from build123d import *

# Parameters (mm, degrees)
BOSS_EXTRUDE1_DEPTH = 4
BOSS_EXTRUDE2_DEPTH = 4
BOSS_EXTRUDE3_DEPTH = 4
SKETCH5_R           = 3
CUT_EXTRUDE2_DEPTH  = 4
SKETCH6_R           = 3
CUT_EXTRUDE3_DEPTH  = 4
SKETCH7_R           = 3
CUT_EXTRUDE4_DEPTH  = 4


with BuildPart() as part:
    # Sketch1 → Boss-Extrude1 (new body)
    with BuildSketch(Plane(origin=(0, 0, 0), x_dir=(1, 0, 0), z_dir=(0, 1, 0))):
        Polygon((0, 0), (160, 0), (160, 37), (37, 37), (37, 160), (0, 160), align=None)
    extrude(amount=BOSS_EXTRUDE1_DEPTH)

    # Sketch3 → Boss-Extrude2 (add)
    with BuildSketch(Plane.XY):
        Polygon((0, 0), (0, 160), (37, 160), (37, 37), (160, 37), (160, 0), align=None)
    extrude(amount=-BOSS_EXTRUDE2_DEPTH)

    # Sketch4 → Boss-Extrude3 (add)
    with BuildSketch(Plane.ZY):
        Polygon((0, 160), (0, 0), (-160, 0), (-160, 37), (-37, 37), (-37, 160), align=None)
    extrude(amount=-BOSS_EXTRUDE3_DEPTH)

    # Sketch5 → Cut-Extrude2 (cut)
    with BuildSketch(Plane.XZ):
        with Locations(Location((135, -22.5, 0), (0, 0, 270))):
            Circle(SKETCH5_R)
        with Locations(Location((110, -22.5, 0), (0, 0, 270))):
            Circle(SKETCH5_R)
        with Locations(Location((85, -22.5, 0), (0, 0, 270))):
            Circle(SKETCH5_R)
        with Locations(Location((22.5, -135, 0), (0, 0, 270))):
            Circle(SKETCH5_R)
        with Locations(Location((22.5, -110, 0), (0, 0, 270))):
            Circle(SKETCH5_R)
        with Locations(Location((22.5, -85, 0), (0, 0, 270))):
            Circle(SKETCH5_R)
        with Locations(Location((22.5, -60, 0), (0, 0, 270))):
            Circle(SKETCH5_R)
        with Locations(Location((60, -22.5, 0), (0, 0, 270))):
            Circle(SKETCH5_R)
    extrude(amount=-CUT_EXTRUDE2_DEPTH, mode=Mode.SUBTRACT)

    # Sketch6 → Cut-Extrude3 (cut)
    with BuildSketch(Plane.ZY):
        with Locations((-135, 22.5)):
            Circle(SKETCH6_R)
        with Locations((-110, 22.5)):
            Circle(SKETCH6_R)
        with Locations((-85, 22.5)):
            Circle(SKETCH6_R)
        with Locations((-60, 22.5)):
            Circle(SKETCH6_R)
        with Locations((-22.5, 135)):
            Circle(SKETCH6_R)
        with Locations((-22.5, 110)):
            Circle(SKETCH6_R)
        with Locations((-22.5, 85)):
            Circle(SKETCH6_R)
        with Locations((-22.5, 60)):
            Circle(SKETCH6_R)
    extrude(amount=-CUT_EXTRUDE3_DEPTH, mode=Mode.SUBTRACT)

    # Sketch7 → Cut-Extrude4 (cut)
    with BuildSketch(Plane.XY):
        with Locations((22.5, 60)):
            Circle(SKETCH7_R)
        with Locations((22.5, 85)):
            Circle(SKETCH7_R)
        with Locations((22.5, 110)):
            Circle(SKETCH7_R)
        with Locations((22.5, 135)):
            Circle(SKETCH7_R)
        with Locations((60, 22.5)):
            Circle(SKETCH7_R)
        with Locations((85, 22.5)):
            Circle(SKETCH7_R)
        with Locations((110, 22.5)):
            Circle(SKETCH7_R)
        with Locations((135, 22.5)):
            Circle(SKETCH7_R)
    extrude(amount=-CUT_EXTRUDE4_DEPTH, mode=Mode.SUBTRACT)


solid = part.part
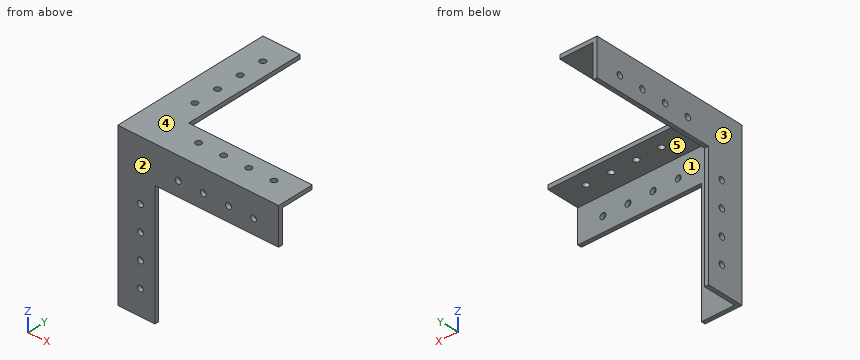
Here's how the part is built. I have some questions about the finished solid (model axes, mm). Face numbers are marked on the shaded views. A direction names the side the tool comes from. Coordinates: 2 decimals unless noted, no trailing zeros. Write each loop counter-clockwise with the first axis right and the second up, starting at its lowest first coordinate (ties: lowest second). Pieces come first, ordered by that corner, then holes.
1) If we section it at B-B (y = 110): List the corners of the cut face in (x, z) for me, plus the area to 3 significant figures.
Filled in:
outline: (0, -37) - (4, -37) - (4, -25.5) - (0, -25.5) - close; (0, -19.5) - (4, -19.5) - (4, -4) - (19.5, -4) - (19.5, 0) - (0, 0) - close; (25.5, -4) - (37, -4) - (37, 0) - (25.5, 0) - close
area: 232 mm2
2) If we section it at D-D (y = 22.5): Count the separate pieces of the cut face and the enclosed holes in it, plus the area to 3 significant figures.
Filled in:
separate pieces: 9
enclosed holes: 0
area: 1,070 mm2
3) Which directions (+Z, -Z, +X, -X, +Y, -Y) give clear straight access to the entire face, cutting with the end or side of a thin tool? Please do the marked faces 1 and 2.
Filled in:
face 1: -Z, +X, +Y
face 2: +Z, -Z, +X, -X, -Y
4) If I drill on line 1 (Y direction, x = 2, z = -22); line 2 (X direction, y = 1.6, z = -22.5); line 3 (Z direction, x = 22, y = 1), over which ranges is the centre line in solid material (lowest first)?
Filled in:
line 1: y = 0 to 57.04, 62.96 to 82.04, 87.96 to 107.04, 112.96 to 132.04, 137.96 to 160
line 2: x = 0 to 57, 63 to 82, 88 to 107, 113 to 132, 138 to 160
line 3: z = -160 to -137.96, -132.04 to -112.96, -107.04 to -87.96, -82.04 to -62.96, -57.04 to 0
5) If we section it at A-A (z = -110): List the corners of the cut face in (x, y) for me, plus the area to 3 significant figures.
Filled in:
outline: (0, 0) - (19.5, 0) - (19.5, 4) - (4, 4) - (4, 19.5) - (0, 19.5) - close; (0, 25.5) - (4, 25.5) - (4, 37) - (0, 37) - close; (25.5, 0) - (37, 0) - (37, 4) - (25.5, 4) - close
area: 232 mm2
6) I'm going to push flat-ended pins straight in: pin 1 (7 mm diameter, centred on x = 22.5, y = 85, fed in from -Z); pin 2 (3.5 mm diameter, centred on y = 22.5, z = -135, fed in from -X); pin 3 (2 mm diameter, centred on y = 1.5, z = -110.5, fed in from +X); pin 4 (9.5 mm diameter, centred on y = 22.5, z = -60, fed in from -X). Where does each tip first touch, or does it pass through?
Filled in:
pin 1: stops at z = -4
pin 2: passes through
pin 3: stops at x = 37
pin 4: stops at x = 0
7) Thinking about a two-plate mould opening in Z: for the marked faces 3, 4 and 5, which applies, +Z half, -Z half, draft (parallel to the pull), parting line (faces both ways), or undercut?
Filled in:
face 3: draft
face 4: +Z half
face 5: -Z half
8) If we section it at C-C (x = 15): List the corners of the cut face in (y, z) for me.
Filled in:
outline: (0, -160) - (4, -160) - (4, -4) - (160, -4) - (160, 0) - (0, 0) - close
